For this review, take the finished solid that the model builds, in its own axes (mm). Face numbers are marked on the shaded views. A direction names the side the tool comes from. Give positions to 0.01 mm unless a question says otherwise; leave off trailing zeros. Order: outer loops, then holes, each group sorted by start corner. A loop starts at its lowest first (then second) coordinate and runs counter-clockwise, first axis right, second up. Notation, with made-up numbers: (10.5, 45.25) - (49.5, 45.25) arc R29 ccw to (49.5, 84.25) - close; hole circle Ø11 at (63.5, -34.5). An arc over 180 degrees is marked (long way). Put each result on its own line as item: value. Start each with the question number.
Autodesk Inventor part; units mm, degrees
ref_plane "YZ Plane" through (0, 0, 0) normal (1, 0, 0) x (0, 1, 0)
ref_plane "XZ Plane" through (0, 0, 0) normal (0, 1, 0) x (-1, 0, 0)
ref_plane "XY Plane" through (0, 0, 0) normal (0, 0, 1) x (1, 0, 0)
sketch "Sketch1" plane through (0, 0, 0) normal (0, 0, 1) x (1, 0, 0)
  line L0 (0, 0) -> (65, 0)
  line L1 (65, 0) -> (65, 8)
  line L2 (65, 8) -> (0, 8)
  line L3 (0, 8) -> (0, 0)
  dimension "d0" = 8
  dimension "d1" = 65
extrude "Extrusion1" add sketch "Sketch1" along normal blind 6.5
sketch "Sketch2" plane through (0, 0, 6.5) normal (0, 0, 1) x (1, 0, 0)
  line L0 (0, 0) -> (65, 0)
  line L1 (65, 8) -> (0, 8)
  line L2 (0, 8) -> (0, 0)
  line L3 (15, 0) -> (23, 0)
  line L4 (23, 0) -> (23, -4.5)
  line L5 (21, -6.5) -> (17, -6.5)
  line L6 (15, -4.5) -> (15, 0)
  line L7 (53, 0) -> (61, 0)
  line L8 (61, 0) -> (61, -4.5)
  line L9 (59, -6.5) -> (55, -6.5)
  line L10 (53, -4.5) -> (53, 0)
  line L11 (8, 8) -> (16, 8)
  line L12 (16, 8) -> (16, 12.5)
  line L13 (14, 14.5) -> (10, 14.5)
  line L14 (8, 12.5) -> (8, 8)
  line L15 (54, 8) -> (62, 8)
  line L16 (62, 8) -> (62, 12.5)
  line L17 (60, 14.5) -> (56, 14.5)
  line L18 (54, 12.5) -> (54, 8)
  arc A0 (15, -4.5) -> (17, -6.5) centre (17, -4.5) ccw
  arc A1 (21, -6.5) -> (23, -4.5) centre (21, -4.5) ccw
  arc A2 (10, 14.5) -> (8, 12.5) centre (10, 12.5) ccw
  arc A3 (16, 12.5) -> (14, 14.5) centre (14, 12.5) ccw
  arc A4 (56, 14.5) -> (54, 12.5) centre (56, 12.5) ccw
  arc A5 (62, 12.5) -> (60, 14.5) centre (60, 12.5) ccw
  arc A6 (53, -4.5) -> (55, -6.5) centre (55, -4.5) ccw
  arc A7 (59, -6.5) -> (61, -4.5) centre (59, -4.5) ccw
  dimension "d4" = 2
  dimension "d5" = 8
  dimension "d6" = 6.5
  dimension "d7" = 6.5
  dimension "d8" = 8
  dimension "d9" = 8
  dimension "d10" = 8
  dimension "d11" = 15
  dimension "d12" = 30
  dimension "d13" = 8
  dimension "d14" = 38
extrude "Extrusion2" add sketch "Sketch2" against normal blind 6.5
properties part number "x_motor_smooth_rod_spacer" material "Plywood, Finish"
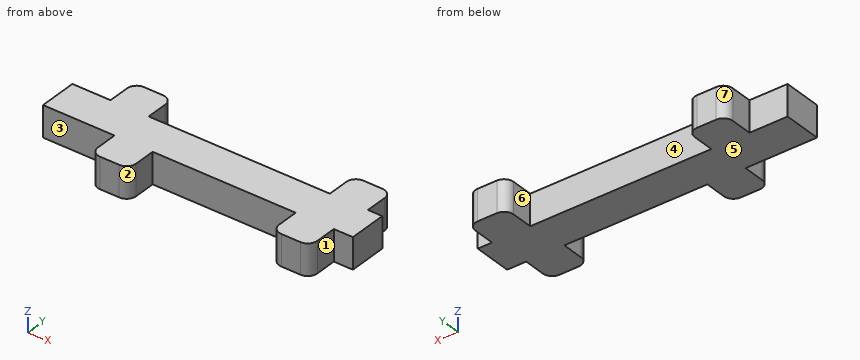
1. Tool access review of the marked faces 1, 2, 3 and 4: name each direction out of +Z, -Z, +X, -X, +Y, -Y from which nothing blocks a thin tool from reaching the whole face with its end or side.
2. Add section A-A, the plane y = 9.5. Give the boundary of the cut face in (x, z), then the cut area to 3 significant figures.
3. Clearance check with flat-ended pins moving along their axes: pin 1 (3.5 mm diameter, centred on y = 11, z = 2.5, fed in from +X); pin 2 (3 mm diameter, centred on x = 9, z = 4, fed in from -Y); pin 3 (1.3 mm diameter, centred on y = -3.5, z = 2.5, fed in from +X); pin 4 (3 mm diameter, centred on x = 55, y = -1.5, fed in from -Z). State where each tip first meets the part, or that it passes through.
4. Add section B-B, the plane z = 3.25. Give the boundary of the cut face in (x, y).
5. Add section D-D, the plane x = 13. Give the boundary of the cut face in (y, z).
6. Wall thickness on line 1 (X direction, y = 10.25, z = 4.75); line 2 (X direction, y = -3, z = 4.5); line 3 (Y direction, x = 19, z = 1.75): over which ranges is each line inside the solid? List them lowest first. Write a range as from..to.
7. Add section C-C, the plane x = 30. Give the boundary of the cut face in (y, z), then the cut area to 3 significant figures.
8. The part is to be moulded in two halves that separate along X. For the marked faces 5, 6 and 7, say which applies: released by +X, released by -X, zero draft, split by the parting line, or undercut.
Found:
1. face 1: +Z, -Z, +X, -Y
1. face 2: +Z, -Z, -Y
1. face 3: +Z, -Z, -X, -Y
1. face 4: +Z, -Z, +Y
2. outline: (8, 0) - (16, 0) - (16, 6.5) - (8, 6.5) - close; (54, 0) - (62, 0) - (62, 6.5) - (54, 6.5) - close
2. area: 104 mm^2
3. pin 1: stops at x = 62
3. pin 2: stops at y = 0
3. pin 3: stops at x = 61
3. pin 4: stops at z = 0
4. outline: (0, 0) - (15, 0) - (15, -4.5) arc R2 ccw to (17, -6.5) - (21, -6.5) arc R2 ccw to (23, -4.5) - (23, 0) - (53, 0) - (53, -4.5) arc R2 ccw to (55, -6.5) - (59, -6.5) arc R2 ccw to (61, -4.5) - (61, 0) - (65, 0) - (65, 8) - (62, 8) - (62, 12.5) arc R2 ccw to (60, 14.5) - (56, 14.5) arc R2 ccw to (54, 12.5) - (54, 8) - (16, 8) - (16, 12.5) arc R2 ccw to (14, 14.5) - (10, 14.5) arc R2 ccw to (8, 12.5) - (8, 8) - (0, 8) - close
5. outline: (0, 0) - (14.5, 0) - (14.5, 6.5) - (0, 6.5) - close
6. line 1: x = 8..16, 54..62
6. line 2: x = 15..23, 53..61
6. line 3: y = -6.5..8
7. outline: (0, 0) - (8, 0) - (8, 6.5) - (0, 6.5) - close
7. area: 52.0 mm^2
8. face 5: zero draft
8. face 6: undercut
8. face 7: released by -X
